The model under review builds one solid part; all positions refer to its coordinate system, in mm. A direction names the side the tool comes from. Round coordinates to 2 decimals unless told otherwise and drop trailing zeros. Write each loop counter-clockwise with the first axis right and the second up, starting at its lowest first coordinate (ties: lowest second). Pieces come first, ordered by that corner, then holes. Notation, with made-up numbers: M 28.5,52.5 L 75.5,52.5 A20 ccw 75.5,82.5 Z; hole C 83,-8.75 d11. An arc over 180 degrees is marked long. One line per item, written item: value. Start each with the question number.
1) Wall thickness on probe 1 along Z at (x, y) = (12.5, 12.5); probe 2 along X at (y, z) = (15.5, -6.5): over which ranges is each line inside the solid? List them lowest first.
2) Take a section at B-B, the plane y = 9. Write out the cut boundary in (x, z).
3) For P1, Ø1, axis at x = -7.5, z = 20, coming from the +Y side; P2, Ø12, axis at y = 16.5, z = -31.5, coming from the -X side; P3, Ø13.5, axis at x = -73.5, y = 31.5, coming from the -Z side, all flat-tipped, find the tip position at first contact; note any pin that passes through.
4) Take a section at D-D, the plane x = 6. Write out the cut boundary in (y, z), and give its area (3 significant figures).
5) Tool access review of faces 4 (the face through (-82, 26, -57.5)), 5 (the face through (82, 26, -57.5)), 6 (the face through (82, 26, 57.5)), 7 (the face through (-1, 5, -1)), 8 (the face through (80.97, 24.43, 0.8)): name each direction out of +Z, -Z, +X, -X, +Y, -Y from which nothing blocks a thin tool from reaching the whole face with its end or side.
6) Mouldability with a two-part tool opening along X and no side actions: class faces 1 (the face through (58, 22, 1)), 2 (the face through (-81.13, 27.8, 0.8)), 3 (the face through (-82, 26, 57.5)) as +X half, -X half, draft (parallel to the pull), parting line (faces both ways), or undercut.
7) Take a section at C-C, the plane y = 23.5. Write out the cut boundary in (x, z), and give its area (3 significant figures).
8) Take a section at A-A, the plane z = -41.5. Write out the cut boundary in (x, y), and give its area (3 significant figures).
from build123d import *

# Parameters (mm, degrees)
SKETCH1_W           = 120
SKETCH1_H           = 120
BOSS_EXTRUDE1_DEPTH = 5
SKETCH1_3_W         = 120
SKETCH1_3_H         = 120
SKETCH1_3_W_2       = 116
SKETCH1_3_H_2       = 116
BOSS_EXTRUDE2_DEPTH = 40
BOSS_EXTRUDE3_DEPTH = 57.5


with BuildPart() as part:
    # Sketch1 → Boss-Extrude1 (new body)
    with BuildSketch(Plane(origin=(0, 0, 0), x_dir=(1, 0, 0), z_dir=(0, 1, 0))):
        Rectangle(SKETCH1_W, SKETCH1_H)
    extrude(amount=BOSS_EXTRUDE1_DEPTH)

    # Sketch1<3> → Boss-Extrude2 (add)
    with BuildSketch(Plane(origin=(0, 0, 0), x_dir=(1, 0, 0), z_dir=(0, 1, 0))):
        Rectangle(SKETCH1_3_W, SKETCH1_3_H)
        Rectangle(SKETCH1_3_W_2, SKETCH1_3_H_2, mode=Mode.SUBTRACT)
    extrude(amount=BOSS_EXTRUDE2_DEPTH)

    # Sketch2 → Boss-Extrude3 (add, symmetric)
    with BuildSketch(Plane.XY):
        Polygon((60, 40), (102.868257487, 15.25), (101.368257487, 12.651923789), (60, 36.535898385), align=None)
    boss_extrude3 = extrude(amount=BOSS_EXTRUDE3_DEPTH, both=True)

    # Mirror1: Boss-Extrude3 across plane
    add(boss_extrude3.mirror(Plane(origin=(0, 0, 0), x_dir=(0, 0, 1), z_dir=(1, 0, 0))))


solid = part.part
Checked values:
1. probe 1: z = -60 to -58, 58 to 60
1. probe 2: x = -102.44 to -96.44, -60 to -58, 58 to 60, 96.44 to 102.44
2. outline: M -60,-60 L 60,-60 L 60,60 L -60,60 Z; hole M -58,-58 L 58,-58 L 58,58 L -58,58 Z
3. P1: stops at y = 5
3. P2: stops at x = -102.87
3. P3: stops at z = -57.5
4. outline: M 0,-60 L 40,-60 L 40,-58 L 5,-58 L 5,58 L 40,58 L 40,60 L 0,60 Z
4. area: 740 mm2
5. face 4: -Z, -X, +Y, -Y
5. face 5: -Z, +X, +Y, -Y
5. face 6: +Z, +X, +Y, -Y
5. face 7: +Y
5. face 8: +Z, -Z, -Y
6. face 1: undercut
6. face 2: -X half
6. face 3: draft
7. outline: M -88.58,-57.5 L -82.58,-57.5 L -82.58,57.5 L -88.58,57.5 Z; M -60,-60 L 60,-60 L 60,60 L -60,60 Z; M 82.58,-57.5 L 88.58,-57.5 L 88.58,57.5 L 82.58,57.5 Z; hole M -58,-58 L 58,-58 L 58,58 L -58,58 Z
7. area: 2,320 mm2
8. outline: M -102.87,15.25 L -101.37,12.65 L -60,36.54 L -60,0 L 60,0 L 60,36.54 L 101.37,12.65 L 102.87,15.25 L 60,40 L 58,40 L 58,5 L -58,5 L -58,40 L -60,40 Z
8. area: 1,030 mm2
